Input: part model. Units: mm. Frame: model coordinates. Coordinates: 2 decimals unless noted, no trailing zeros. Write each loop counter-clockwise with the first axis right and the second up, starting at its lowest first coordinate (ties: lowest second). Pieces come first, ordered by that corner, then holes. Notation, with made-up numbers: M -30,37 L 6,37 A13 ccw 6,59 Z; hole C 22.25,-0.75 d6. An arc over 180 degrees is marked long. Write each question's results on one line, items separated by ' | '. Start each with the question number.
1. Section query C-C, the plane y = 7. Count the separate pieces of the cut face and the enclosed holes in it, and give its area (3 significant figures).
2. First-contact query: pin 1 (2 mm diameter, centred on x = -279, y = 5, fed in from +Z). Flat tip, straight axial feed; report the tip coordinate or a pass-through.
3. Section query A-A, the plane z = -395. Output: boundary loops of the cut face in (x, y).
4. Section query B-B, the plane x = -223. Output: boundary loops of the cut face in (y, z), and give its area (3 significant figures).
5. Ray query, probe 1 along X at (y, z) = (2.75, -158.5); probe 2 along Z at (x, y) = (-197, 0.5); probe 3 along Z at (x, y) = (-92.5, 8.25). Return the intervals inside material, ascending.
Autodesk Inventor part; units mm, degrees
ref_plane "YZ Plane" through (0, 0, 0) normal (1, 0, 0) x (0, 1, 0)
ref_plane "XZ Plane" through (0, 0, 0) normal (0, 1, 0) x (-1, 0, 0)
ref_plane "XY Plane" through (0, 0, 0) normal (0, 0, 1) x (1, 0, 0)
sketch "Sketch1" plane through (0, 0, 0) normal (0, 1, 0) x (-1, 0, 0)
  line L0 (75.2406, 23.4715) -> (252.2406, 23.4715)
  line L1 (382.2406, -68.5285) -> (382.2406, -499.5285)
  line L2 (252.2406, -591.5285) -> (75.2406, -591.5285)
  line L3 (-54.7594, -499.5285) -> (-54.7594, -68.5285)
  line L4 (-54.7594, -284.0285) -> (382.2406, -284.0285)
  line L5 (382.2406, -284.0285) -> (382.2406, -499.5285)
  line L6 (163.7406, 23.4715) -> (163.7406, -591.5285)
  line L7 (163.7406, -591.5285) -> (252.2406, -591.5285)
  line L8 (252.2406, -591.5285) -> (382.2406, -499.5285)
  line L9 (75.2406, -591.5285) -> (-54.7594, -499.5285)
  line L10 (252.2406, 23.4715) -> (382.2406, -68.5285)
  line L11 (75.2406, 23.4715) -> (-54.7594, -68.5285)
  point P0 (0, 0)
  dimension "d0" = 437
  dimension "d2" = 215.5
  dimension "d3" = 88.5
  dimension "d4" = 615
extrude "Extrusion1" add sketch "Sketch1" along normal blind 10
sketch "Sketch2" plane through (0, 10, 0) normal (0, 1, 0) x (1, 0, 0)
  line L0 (-382.2406, 499.5285) -> (-382.2406, 68.5285)
  line L1 (-252.2406, -23.4715) -> (-75.2406, -23.4715)
  line L2 (-75.2406, -23.4715) -> (54.7594, 68.5285)
  line L3 (54.7594, 68.5285) -> (54.7594, 499.5285)
  line L4 (54.7594, 499.5285) -> (-75.2406, 591.5285)
  line L5 (-75.2406, 591.5285) -> (-252.2406, 591.5285)
  line L6 (-163.7406, 591.5285) -> (-163.7406, -23.4715)
  line L7 (-382.2406, 499.5285) -> (54.7594, 499.5285)
  line L8 (-163.7406, 499.5285) -> (-90.7406, 499.5285)
  line L9 (-90.7406, 499.5285) -> (39.2594, 499.5285)
  line L10 (39.2594, 499.5285) -> (39.2594, 510.4977)
  line L11 (-382.2406, 284.0285) -> (54.7594, 284.0285)
  circle A0 centre (39.2594, 284.0285) radius 2.5
  line L12 (39.2594, 284.0285) -> (39.2594, 357.0285)
  line L13 (39.2594, 359.5285) -> (39.2594, 430.0285)
  circle A1 centre (39.2594, 357.0285) radius 2.5
  circle A2 centre (39.2594, 211.0285) radius 2.5
  circle A3 centre (-366.7406, 357.0285) radius 2.5
  circle A4 centre (-366.7406, 211.0285) radius 2.5
  line L14 (39.2594, 393.5285) -> (-90.7406, 393.5285)
  line L15 (-90.7406, 393.5285) -> (-90.7406, 540.5285)
  circle A5 centre (39.2594, 430.0285) radius 2.5
  line L16 (-90.7406, 430.0285) -> (-90.7406, 576.0285)
  circle A6 centre (-90.7406, 576.0285) radius 2.5
  line L17 (-382.2406, 68.5285) -> (54.7594, 68.5285)
  circle A7 centre (39.2594, 138.0285) radius 2.5
  circle A8 centre (-90.7406, -7.9715) radius 2.5
  circle A9 centre (-366.7406, 430.0285) radius 2.5
  circle A10 centre (-236.7406, 576.0285) radius 2.5
  circle A11 centre (-236.7406, -7.9715) radius 2.5
  circle A12 centre (-366.7406, 138.0285) radius 2.5
  line L18 (-90.7406, 499.5285) -> (-90.7406, 68.5285)
  line L19 (-90.7406, -23.4715) -> (-90.7406, -34.4408)
  line L20 (-90.7406, 499.5285) -> (-90.7406, 573.5285)
  line L21 (-90.7406, 591.5285) -> (-90.7406, 602.4977)
  line L22 (39.2594, 499.5285) -> (39.2594, 281.5285)
  line L23 (39.2594, 68.5285) -> (39.2594, 57.5592)
  circle A13 centre (-366.7406, 284.0285) radius 2.5
  point P0 (0, 0)
  dimension "d9" = 5
  dimension "d12" = 5
  dimension "d22" = 5
  dimension "d7" = 73
  dimension "d8" = 130
  dimension "d10" = 73
  dimension "d11" = 73
  dimension "d19" = 5
  dimension "d20" = 615
  dimension "d21" = 146
  dimension "d23" = 437
  dimension "d25" = 5
extrude "Extrusion2" cut sketch "Sketch2" against normal blind 10 contours A6 | A13 L11 | L11 A13 | A0 L12 L11 | L11 L22 A0 | L22 L13 A5 | A5 L13 L22 | L12 A0 L11 | L11 A0 L22 | A1 L22 L12 | L12 L22 A1 | A2 | A3 | A4 | A7 | A8 | A9 | A10 | A11 | A12
sketch "Sketch3" plane through (0, 10, 0) normal (0, 1, 0) x (1, 0, 0)
  line L0 (-382.2406, 499.5285) -> (-382.2406, 68.5285)
  line L1 (-382.2406, 68.5285) -> (-252.2406, -23.4715)
  line L2 (-252.2406, -23.4715) -> (-75.2406, -23.4715)
  line L3 (-75.2406, -23.4715) -> (54.7594, 68.5285)
  line L4 (54.7594, 68.5285) -> (54.7594, 499.5285)
  line L5 (54.7594, 499.5285) -> (-75.2406, 591.5285)
  line L6 (-75.2406, 591.5285) -> (-252.2406, 591.5285)
  line L7 (-252.2406, 591.5285) -> (-382.2406, 499.5285)
  line L8 (-85.1002, 560.5285) -> (23.7594, 483.4894)
  line L9 (23.7594, 483.4894) -> (23.7594, 84.5676)
  line L10 (23.7594, 84.5676) -> (-85.1002, 7.5285)
  line L11 (-85.1002, 7.5285) -> (-242.381, 7.5285)
  line L12 (-242.381, 7.5285) -> (-351.2406, 84.5676)
  line L13 (-351.2406, 84.5676) -> (-351.2406, 483.4894)
  line L14 (-351.2406, 483.4894) -> (-242.381, 560.5285)
  line L15 (-242.381, 560.5285) -> (-85.1002, 560.5285)
  line L16 (-382.2406, 319.1066) -> (-351.2406, 319.1066)
  point P0 (0, 0)
  dimension "d26" = 31
extrude "Extrusion3" cut sketch "Sketch3" against normal blind 10 contours L13 L14 L15 L8 L9 L10 L11 L12
properties part number "mount_holes_plate"
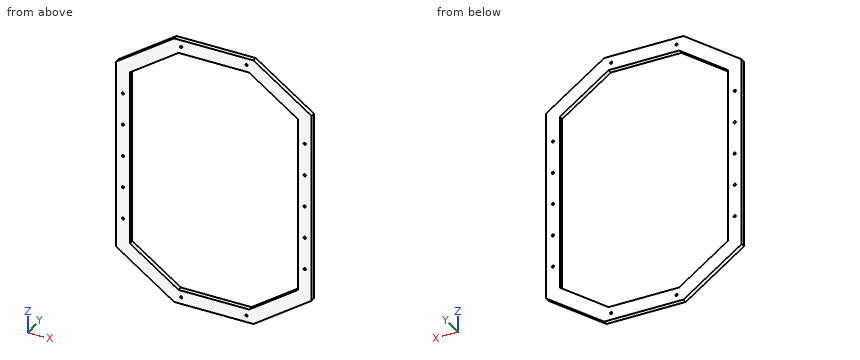
Answer:
1) separate pieces: 1 | enclosed holes: 15 | area: 54,000 mm^2
2) pin 1: z = 5.24
3) outline: M -382.24,0 L -351.24,0 L -351.24,10 L -382.24,10 Z; M 23.76,0 L 54.76,0 L 54.76,10 L 23.76,10 Z
4) outline: M 0,-591.53 L 10,-591.53 L 10,-560.53 L 0,-560.53 Z; M 0,-7.53 L 10,-7.53 L 10,23.47 L 0,23.47 Z | area: 620 mm^2
5) probe 1: -382.24 to -351.24, 23.76 to 54.76 | probe 2: -591.53 to -560.53, -7.53 to 23.47 | probe 3: -591.53 to -577.8, -574.25 to -560.53, -7.53 to 6.2, 9.75 to 23.47
